from build123d import *

# Parameters (mm, degrees)
FILLET1_R = 1


with BuildPart() as part:
    # Sketch3 → Revolve1 (revolve)
    with BuildSketch(Plane.XY, mode=Mode.PRIVATE) as revolve1_sk:
        Polygon((6, 15), (-6, 15), (-6, 20), (-5.3, 20), (-5.3, 30), (-6, 30), (-6, 35.5), (6, 35.5), (6, 30), (5.3, 30), (5.3, 20), (6, 20), align=None)
    revolve(revolve1_sk.sketch.rotate(Axis((-14.54061226, 0, 0), (1, 0, 0)), 90), axis=Axis((-14.54061226, 0, 0), (1, 0, 0)))

    # Fillet1
    # the kernel refuses this fillet: 1 mm, written as the material it adds along each edge
    with BuildSketch(Plane(origin=(5.3, 0, 0), x_dir=(0, 0, 1), z_dir=(0, 1, 0))) as fillet1_piece_1:
        with BuildLine():
            CenterArc((29.046060799, 1), FILLET1_R, 270, 72.542396876)
            Line((29.046060799, 0), (29.046060799, -0.02))
            Line((29.046060799, -0.02), (30, -0.02))
            Line((30, -0.02), (30.02, 0))
            ThreePointArc((30.02, 0), (30.02, 0.35), (30.019078784, 0.694))
            Line((30.019078784, 0.694), (30, 0.7))
        make_face()
    revolve(axis=Axis((5.3, 0, 0), (1, 0, 0)))
    with BuildSketch(Plane(origin=(-5.3, 0, 0), x_dir=(0, 0, 1), z_dir=(0, 1, 0))) as fillet1_piece_2:
        with BuildLine():
            CenterArc((29.046060799, -1), FILLET1_R, 17.457603124, 72.542396876)
            Line((30, -0.7), (30.019078784, -0.694))
            ThreePointArc((30.019078784, -0.694), (30.02, -0.35), (30.02, 0))
            Line((30.02, 0), (30, 0.02))
            Line((30, 0.02), (29.046060799, 0.02))
            Line((29.046060799, 0.02), (29.046060799, 0))
        make_face()
    revolve(axis=Axis((-5.3, 0, 0), (1, 0, 0)))
    # the kernel refuses this fillet: 1 mm, written as the material it takes off along each edge
    with BuildSketch(Plane(origin=(6, 0, 0), x_dir=(0, 0, 1), z_dir=(0, 1, 0))) as fillet1_2_piece_1:
        with BuildLine():
            CenterArc((19.046060799, -1), FILLET1_R, 17.457603124, 72.542396876)
            Line((20, -0.7), (20.019078784, -0.694))
            ThreePointArc((20.019078784, -0.694), (20.02, -0.35), (20.02, 0))
            Line((20.02, 0), (20, 0.02))
            Line((20, 0.02), (19.046060799, 0.02))
            Line((19.046060799, 0.02), (19.046060799, 0))
        make_face()
    revolve(axis=Axis((6, 0, 0), (1, 0, 0)), mode=Mode.SUBTRACT)
    with BuildSketch(Plane(origin=(-6, 0, 0), x_dir=(0, 0, 1), z_dir=(0, 1, 0))) as fillet1_2_piece_2:
        with BuildLine():
            CenterArc((19.046060799, 1), FILLET1_R, 270, 72.542396876)
            Line((20, 0.7), (20.019078784, 0.694))
            ThreePointArc((20.019078784, 0.694), (20.02, 0.35), (20.02, 0))
            Line((20.02, 0), (20, -0.02))
            Line((20, -0.02), (19.046060799, -0.02))
            Line((19.046060799, -0.02), (19.046060799, 0))
        make_face()
    revolve(axis=Axis((-6, 0, 0), (1, 0, 0)), mode=Mode.SUBTRACT)


solid = part.part
Verification items for the finished model (mm, model axes). A direction names the side the tool comes from. Give positions to 0.01 mm unless a question says otherwise; leave off trailing zeros. Order: outer loops, then holes, each group sorted by start corner. A loop starts at its lowest first (then second) coordinate and runs counter-clockwise, first axis right, second up. Notation, with made-up numbers: (73.25, 68.25) -> (100.25, 68.25) arc R20 ccw to (100.25, 101.25) -> close; hole circle Ø3 at (65.25, 16). An arc over 180 degrees is marked (long way). Answer as CSV lines item,"result".
Q1. Depth check by flat-ended pin: pin 1 (6 mm diameter, centred on x = -3, z = 0.5, fed in from +Y); pin 2 (4 mm diameter, centred on x = -1.5, z = 8, fed in from -Y); pin 3 (5 mm diameter, centred on x = -2, z = 24.5, fed in from +Y). Enter the tip coordinate at first touch or a pass-through.
Solutions:
pin 1,"stops at y = 35.5"
pin 2,"stops at y = -34.99"
pin 3,"stops at y = 27.86"
Q2. Sectioned sample at C-C on x = -2.25. Record the cut outline in (y, z), plus the area to 3 significant figures.
Solutions:
outline,"circle Ø71 at (0, 0); hole circle Ø30 at (0, 0)"
area,"3,250 mm²"
Q3. Scan lines: probe 1 along Y at (x, z) = (0.5, 0); probe 2 along Z at (x, y) = (-0.75, -10); probe 3 along X at (y, z) = (-18.5, 18.5). Record each from-to range of solid material in increasing order.
Solutions:
probe 1,"y = -35.5 to -15, 15 to 35.5"
probe 2,"z = -34.06 to -11.18, 11.18 to 34.06"
probe 3,"x = -5.3 to 5.3"
Q4. Release check for a two-part mould opening along Y. For faces 4 (the cylindrical face through (-0.08, -12.65, 8.06)), 5 (the cylindrical face through (0.084, 34.656, -7.696)), 6 (the flat face through (-6, 14, -6)) record: +Y half, -Y half, draft (parallel to the pull), parting line (faces both ways), or undercut.
Solutions:
face 4,"undercut"
face 5,"parting line"
face 6,"draft"
Q5. Access from +Z, -Z, +X, -X, +Y, -Y to the whole of each face (thin tool, end or side, straight path). Record for faces 1 (the flat face through (-5.3, -7, -19)), 2 (the flat face through (6, 14, 6)), 3 (the flat face through (5.3, -7, 19)).
Solutions:
face 1,"-X"
face 2,"+Z, -Z, +X, +Y, -Y"
face 3,"+X"
Q6. Sectioned sample at A-A on y = 0. Record the cut outline in (x, z), plus the area to 3 significant figures.
Solutions:
outline,"(-6, -35.5) -> (6, -35.5) -> (6, -30) arc R1 cw to (5.3, -29.05) -> (5.3, -20) arc R1 ccw to (6, -19.05) -> (6, -15) -> (-6, -15) -> (-6, -19.05) arc R1 ccw to (-5.3, -20) -> (-5.3, -29.05) arc R1 cw to (-6, -30) -> close; (-6, 15) -> (6, 15) -> (6, 19.05) arc R1 ccw to (5.3, 20) -> (5.3, 29.05) arc R1 cw to (6, 30) -> (6, 35.5) -> (-6, 35.5) -> (-6, 30) arc R1 cw to (-5.3, 29.05) -> (-5.3, 20) arc R1 ccw to (-6, 19.05) -> close"
area,"464 mm²"
